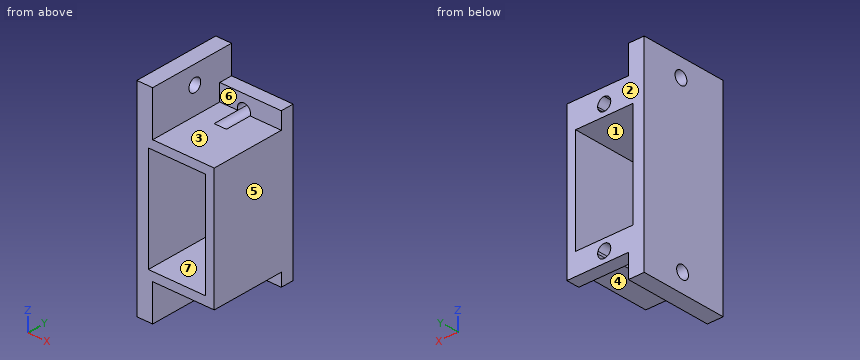
from build123d import *

# Parameters (mm, degrees)
SKETCH1_W               = 13.1
SKETCH1_H               = 24
BOSS_EXTRUDE1_DEPTH     = 20
CUT_EXTRUDE1_DEPTH      = 37.333765723
CUT_EXTRUDE1_DEPTH_BACK = 37.333765723
SKETCH4_R               = 1.5
BOSS_EXTRUDE2_START     = 17
BOSS_EXTRUDE2_DEPTH     = 3
BOSS_EXTRUDE3_DEPTH     = 11


with BuildPart() as part:
    # Sketch1 → Boss-Extrude1 (new body)
    with BuildSketch(Plane(origin=(0, 0, 0), x_dir=(1, 0, 0), z_dir=(0, 1, 0))):
        with BuildLine():
            Line((51.803705275, -9.5), (51.803705275, 18.5))
            Line((51.803705275, 18.5), (44.667918837, 18.5))
            ThreePointArc((44.667918837, 18.5), (43.253705275, 17.5), (41.839491713, 18.5))
            Line((41.839491713, 18.5), (37.703705275, 18.5))
            Line((37.703705275, 18.5), (37.703705275, 26.857634512))
            Line((37.703705275, 26.857634512), (34.090699836, 26.857634512))
            Line((34.090699836, 26.857634512), (34.090699836, -19.776172663))
            Line((34.090699836, -19.776172663), (37.703705275, -19.776172663))
            Line((37.703705275, -19.776172663), (37.703705275, -9.5))
            Line((37.703705275, -9.5), (41.839491713, -9.5))
            ThreePointArc((41.839491713, -9.5), (43.253705275, -8.5), (44.667918837, -9.5))
            Line((44.667918837, -9.5), (51.803705275, -9.5))
        make_face()
        with Locations((43.253705275, 4.5)):
            Rectangle(SKETCH1_W, SKETCH1_H, mode=Mode.SUBTRACT)
    extrude(amount=BOSS_EXTRUDE1_DEPTH)

    # Sketch4 → Cut-Extrude1 (cut, two sides: drawn at the far end of the back side and taken through both)
    with BuildSketch(Plane(origin=(37.703705275, 0, 0), x_dir=(0, 0, -1), z_dir=(1, 0, 0)).offset(-CUT_EXTRUDE1_DEPTH_BACK)):
        with Locations((-15.603546026, 10.694249846)):
            Circle(SKETCH4_R)
        with Locations(Location((22.568421885, 10.286160732, 0), (0, 0, 180))):
            Circle(SKETCH4_R)
    extrude(amount=CUT_EXTRUDE1_DEPTH + CUT_EXTRUDE1_DEPTH_BACK, mode=Mode.SUBTRACT)

    # Sketch1<31> → Boss-Extrude2 (add)
    with BuildSketch(Plane(origin=(0, 0, 0), x_dir=(1, 0, 0), z_dir=(0, 1, 0)).offset(BOSS_EXTRUDE2_START)):
        with BuildLine():
            Line((51.803705275, -13.351943518), (51.803705275, -9.5))
            Line((51.803705275, -9.5), (44.667918837, -9.5))
            ThreePointArc((44.667918837, -9.5), (44.732103114, -9.746347032), (44.753705275, -10))
            ThreePointArc((44.753705275, -10), (44.314365447, -11.060660172), (43.253705275, -11.5))
            Line((43.253705275, -11.5), (43.253705275, -13.351943518))
            Line((43.253705275, -13.351943518), (51.803705275, -13.351943518))
        make_face()
        with BuildLine():
            Line((37.703705275, -13.351943518), (43.253705275, -13.351943518))
            Line((43.253705275, -13.351943518), (43.253705275, -11.5))
            ThreePointArc((43.253705275, -11.5), (42.028960404, -10.866025404), (41.839491713, -9.5))
            Line((41.839491713, -9.5), (37.703705275, -9.5))
            Line((37.703705275, -9.5), (37.703705275, -13.351943518))
        make_face()
        with BuildLine():
            Line((44.667918837, 18.5), (51.803705275, 18.5))
            Line((51.803705275, 18.5), (51.803705275, 21.478401139))
            Line((51.803705275, 21.478401139), (43.253705275, 21.478401139))
            Line((43.253705275, 21.478401139), (43.253705275, 20.5))
            ThreePointArc((43.253705275, 20.5), (44.314365447, 20.060660172), (44.753705275, 19))
            ThreePointArc((44.753705275, 19), (44.732103114, 18.746347032), (44.667918837, 18.5))
        make_face()
        with BuildLine():
            Line((43.253705275, 20.5), (43.253705275, 21.478401139))
            Line((43.253705275, 21.478401139), (37.703705275, 21.478401139))
            Line((37.703705275, 21.478401139), (37.703705275, 18.5))
            Line((37.703705275, 18.5), (41.839491713, 18.5))
            ThreePointArc((41.839491713, 18.5), (42.028960404, 19.866025404), (43.253705275, 20.5))
        make_face()
    extrude(amount=BOSS_EXTRUDE2_DEPTH)

    # Sketch1<32> → Boss-Extrude3 (add)
    with BuildSketch(Plane(origin=(0, 0, 0), x_dir=(1, 0, 0), z_dir=(0, 1, 0))):
        with BuildLine():
            Line((44.667918837, 18.5), (41.839491713, 18.5))
            ThreePointArc((41.839491713, 18.5), (43.253705275, 17.5), (44.667918837, 18.5))
        make_face()
        with BuildLine():
            ThreePointArc((44.667918837, -9.5), (43.253705275, -8.5), (41.839491713, -9.5))
            Line((41.839491713, -9.5), (44.667918837, -9.5))
        make_face()
    extrude(amount=BOSS_EXTRUDE3_DEPTH)


solid = part.part
Design review of the part built by this model. Coordinates are the model's own, in mm. Face numbers are marked on the shaded views. A direction names the side the tool comes from. Round coordinates to 2 decimals unless told otherwise and drop trailing zeros. Write each loop counter-clockwise with the first axis right and the second up, starting at its lowest first coordinate (ties: lowest second). Pieces come first, ordered by that corner, then holes. Notation, with made-up numbers: M -20.5,52 L -7.5,52 A33 cw -7.5,82 Z; hole C -14,85 d2. An arc over 180 degrees is marked long. One line per item, written item: value. Start each with the question number.
1. To check wall thickness, follow probe 1 along Z at (x, y) = (39.75, 11); probe 2 along X at (y, z) = (13.25, -15); probe 3 along Z at (x, y) = (36.75, 12.5). State the ranges of each line that lie inside material, in increasing order. Write a range as from..to.
2. For the marked faces 5, 6 and 7, list the 3-axis set-ups (+Z, -Z, +X, -X, +Y, -Y) from which the entire face can be reached by the end or side of a thin tool; tool diameter is ignored.
3. Take a section at A-A on z = -5. State the section outline as (x, y) points, then the cut area to 3 significant figures.
4. Clearance check with flat-ended pins moving along their axes: P1, Ø4, axis at y = 10.29, z = -22.57, coming from the +X side; P2, Ø3.5, axis at x = 41.5, y = 18, coming from the +Z side; P3, Ø1, axis at x = 41, y = 3.5, coming from the -Z side; P4, Ø10.5, axis at x = 42, y = 9.5, coming from the +Z side. State where each tip first meets the part, or that it passes through.
5. Take a section at D-D on x = 50.5. State the section outline as (y, z) points, then the cut area to 3 significant figures.
6. Take a section at C-C on y = 16.5. State the section outline as (x, z) points.
7. Draft analysis for pull direction Z (two halves, no side actions). For the marked faces 1, 2, 3 and 4, state which applies: pulls with the +Z half, pulls with the -Z half, needs draft (parallel to the pull), parting line crosses it, or undercut.
8. Take a section at B-B on x = 40.5. State the section outline as (y, z) points, then the cut area to 3 significant figures.
Computed:
1. probe 1: z = -18.5..-16.5, 7.5..9.5
1. probe 2: x = 34.09..36.7, 49.8..51.8
1. probe 3: z = -26.86..-16.5, 7.5..19.78
2. face 5: +Z, -Z, +X, +Y, -Y
2. face 6: +Z, +X, -Y
2. face 7: +Y, -Y
3. outline: M 34.09,0 L 36.7,0 L 36.7,20 L 34.09,20 Z; M 49.8,0 L 51.8,0 L 51.8,20 L 49.8,20 Z
3. area: 92.3 mm²
4. P1: stops at x = 37.7
4. P2: stops at z = 13.35
4. P3: stops at z = -18.5
4. P4: stops at z = 19.78
5. outline: M 0,-18.5 L 17,-18.5 L 17,-21.48 L 20,-21.48 L 20,13.35 L 17,13.35 L 17,9.5 L 0,9.5 Z
5. area: 580 mm²
6. outline: M 34.09,-26.86 L 37.7,-26.86 L 37.7,-18.5 L 41.84,-18.5 A1.5 cw 44.67,-18.5 L 51.8,-18.5 L 51.8,9.5 L 44.67,9.5 A1.5 cw 41.84,9.5 L 37.7,9.5 L 37.7,19.78 L 34.09,19.78 Z; hole M 36.7,-16.5 L 49.8,-16.5 L 49.8,7.5 L 36.7,7.5 Z
7. face 1: undercut
7. face 2: needs draft
7. face 3: pulls with the +Z half
7. face 4: pulls with the -Z half
8. outline: M 0,-18.5 L 17,-18.5 L 17,-21.48 L 20,-21.48 L 20,-16.5 L 0,-16.5 Z; M 0,7.5 L 20,7.5 L 20,13.35 L 17,13.35 L 17,9.5 L 0,9.5 Z
8. area: 100 mm²
